```python
from build123d import *

# Parameters (mm, degrees)
SKETCH1_R           = 19
SKETCH1_R_2         = 2.1
SKETCH1_R_3         = 7.1
SKETCH1_R_4         = 2
BOSS_EXTRUDE1_DEPTH = 16.25
SKETCH2_R           = 7.6
CUT_EXTRUDE1_DEPTH  = 1.1
SKETCH3_R           = 7.75
CUT_EXTRUDE2_DEPTH  = 1.05
SKETCH4_R           = 2.1
CUT_EXTRUDE3_DEPTH  = 5


with BuildPart() as part:
    # Sketch1 → Boss-Extrude1 (new body)
    with BuildSketch(Plane(origin=(0, 0, 0), x_dir=(1, 0, 0), z_dir=(0, 1, 0))):
        Circle(SKETCH1_R)
        with Locations((-8, 8)):
            Circle(SKETCH1_R_2, mode=Mode.SUBTRACT)
        with Locations((-8, -8)):
            Circle(SKETCH1_R_2, mode=Mode.SUBTRACT)
        with Locations((8, 8)):
            Circle(SKETCH1_R_2, mode=Mode.SUBTRACT)
        with Locations((8, -8)):
            Circle(SKETCH1_R_2, mode=Mode.SUBTRACT)
        Circle(SKETCH1_R_3, mode=Mode.SUBTRACT)
        with Locations((0, 11.315)):
            Circle(SKETCH1_R_4, mode=Mode.SUBTRACT)
        with Locations((11.315, 0)):
            Circle(SKETCH1_R_4, mode=Mode.SUBTRACT)
        with Locations((0, -11.315)):
            Circle(SKETCH1_R_4, mode=Mode.SUBTRACT)
        with Locations((-11.315, 0)):
            Circle(SKETCH1_R_4, mode=Mode.SUBTRACT)
    extrude(amount=BOSS_EXTRUDE1_DEPTH)

    # Sketch2 → Cut-Extrude1 (cut)
    with BuildSketch(Plane(origin=(0, 16.25, 0), x_dir=(1, 0, 0), z_dir=(0, 1, 0))):
        Circle(SKETCH2_R)
    extrude(amount=-CUT_EXTRUDE1_DEPTH, mode=Mode.SUBTRACT)

    # Sketch3 → Cut-Extrude2 (cut)
    with BuildSketch(Plane.XZ):
        Circle(SKETCH3_R)
    extrude(amount=-CUT_EXTRUDE2_DEPTH, mode=Mode.SUBTRACT)

    # Sketch4 → Cut-Extrude3 (cut)
    with BuildSketch(Plane(origin=(0, 16.25, 0), x_dir=(1, 0, 0), z_dir=(0, 1, 0))):
        Polygon((-11.185438763, 8.934779773), (-10.402262411, 5.708718996), (-7.216823649, 4.773939223), (-4.814561237, 7.065220227), (-5.597737589, 10.291281004), (-8.783176351, 11.226060777), align=None)
        with Locations((-8, 8)):
            Circle(SKETCH4_R, mode=Mode.SUBTRACT)
        Polygon((7.216823649, 4.773939223), (4.814561237, 7.065220227), (5.597737589, 10.291281004), (8.783176351, 11.226060777), (11.185438763, 8.934779773), (10.402262411, 5.708718996), align=None)
        with Locations((8, 8)):
            Circle(SKETCH4_R, mode=Mode.SUBTRACT)
        Polygon((-7.216823649, -4.773939223), (-4.814561237, -7.065220227), (-5.597737589, -10.291281004), (-8.783176351, -11.226060777), (-11.185438763, -8.934779773), (-10.402262411, -5.708718996), align=None)
        with Locations((-8, -8)):
            Circle(SKETCH4_R, mode=Mode.SUBTRACT)
        Polygon((11.185438763, -8.934779773), (10.402262411, -5.708718996), (7.216823649, -4.773939223), (4.814561237, -7.065220227), (5.597737589, -10.291281004), (8.783176351, -11.226060777), align=None)
        with Locations((8, -8)):
            Circle(SKETCH4_R, mode=Mode.SUBTRACT)
    extrude(amount=-CUT_EXTRUDE3_DEPTH, mode=Mode.SUBTRACT)


solid = part.part
```
Work out the finished part from the listing and answer in its coordinate system (mm). A direction names the side the tool comes from. Coordinates: 2 decimals unless noted, no trailing zeros. Loops run counter-clockwise (first coordinate to the right, second up) from the corner with the lowest first, then second, coordinate; pieces in that order, holes last. Notation, with made-up numbers: M -3,9.5 L 23,9.5 A31 ccw 23,42.5 Z; hole C -10,0 d11. An arc over 180 degrees is marked long. Use CSV: the item, a comma, the result in double quotes. Start each with the question number.
(1) Find section C-C, the plane y = 9.5. State how many separate pieces and enclosed holes the cut face has, then the cut area to 3 significant figures.
(2) For faces 5 (the face through (13.16, 8.01, 0.77)), 6 (the face through (-2, 15.15, -7)), 7 (the face through (-1.009, 0.518, 7.684)), determine the directions among +Z, -Z, +X, -X, +Y, -Y from which every point of the face is accessible in a straight line to the end or side of a thin tool.
(3) For a pull along Z with two mould halves and no side action, classify faces 1 (the face through (8, 0, 0)), 2 (the face through (-10.8, 13.78, 7.34)), 3 (the face through (8.767, 8.011, 16.856)), 4 (the face through (9.967, 13.785, -10.096)) as +Z half, -Z half, draft (parallel to the pull), parting line (faces both ways), or undercut.
(4) Given pin 1 Ø13 at (x, z) = (0, 0) entering from +Y; pin 2 Ø1.5 at (y, z) = (7, 4.5) entering from -X; pin 3 Ø3 at (x, y) = (-14.5, 9.5) entering from +Z; pin 4 Ø1.5 at (y, z) = (1.5, -10) entering from +X, each flat-ended and moving along its own axis, determine where each tip first touches the part or whether it passes through.
(5) Find section A-A, the plane x = 0. Give the vertices of the cut face in (y, z) (3 decimals).
(6) Find section D-D, the plane z = -17. Give the vertices of the cut face in (x, y), then the cut area to 3 significant figures.
(7) Consider line 1 (X direction, y = 15.65, z = 0) (3 decimals); line 2 (X direction, y = 10.5, z = 9). Determine where each line is inside the solid, lowest interval first.
(8) Find section B-B, the plane z = 0. Give the vertices of the cut face in (x, y) (3 decimals), then the cut area to 3 significant figures.
Recorded:
1,separate pieces,"1"
1,enclosed holes,"9"
1,area,"870 mm^2"
2,face 5,"+Y, -Y"
2,face 6,"+Y"
2,face 7,"-Y"
3,face 1,"draft"
3,face 2,"undercut"
3,face 3,"parting line"
3,face 4,"undercut"
4,pin 1,"passes through"
4,pin 2,"stops at x = -18.63"
4,pin 3,"stops at z = 13.86"
4,pin 4,"stops at x = 16.6"
5,outline,"M 0,-19 L 16.25,-19 L 16.25,-13.315 L 0,-13.315 Z; M 0,-9.315 L 16.25,-9.315 L 16.25,-7.6 L 15.15,-7.6 L 15.15,-7.1 L 1.05,-7.1 L 1.05,-7.75 L 0,-7.75 Z; M 0,7.75 L 1.05,7.75 L 1.05,7.1 L 15.15,7.1 L 15.15,7.6 L 16.25,7.6 L 16.25,9.315 L 0,9.315 Z; M 0,13.315 L 16.25,13.315 L 16.25,19 L 0,19 Z"
6,outline,"M -8.49,0 L 8.49,0 L 8.49,16.25 L -8.49,16.25 Z"
6,area,"276 mm^2"
7,line 1,"x = -19 to -13.315, -9.315 to -7.6, 7.6 to 9.315, 13.315 to 19"
7,line 2,"x = -16.73 to -9.85, -6.15 to 6.15, 9.85 to 16.73"
8,outline,"M -19,0 L -13.315,0 L -13.315,16.25 L -19,16.25 Z; M -9.315,0 L -7.75,0 L -7.75,1.05 L -7.1,1.05 L -7.1,15.15 L -7.6,15.15 L -7.6,16.25 L -9.315,16.25 Z; M 7.1,1.05 L 7.75,1.05 L 7.75,0 L 9.315,0 L 9.315,16.25 L 7.6,16.25 L 7.6,15.15 L 7.1,15.15 Z; M 13.315,0 L 19,0 L 19,16.25 L 13.315,16.25 Z"
8,area,"254 mm^2"
